Study the drawing (mm; zero at the part's minimum x, y, z) and answer. A direction names the side the tool comes from. Give positions to 0.01 mm unless a question says otherwise; leave off trailing zeros. Loops run counter-clockwise (first coordinate to the right, second up) from the corner with the lowest first, then second, coordinate; pieces in that order, holes last. Notation, with made-up numbers: (12, 37.25) - (54, 37.25) arc R31 cw to (54, 76.25) - close; hole circle Ø9 at (-35, -12.75). An arc over 180 degrees is marked (long way). Write item = value, one per line. Start each with the question number.
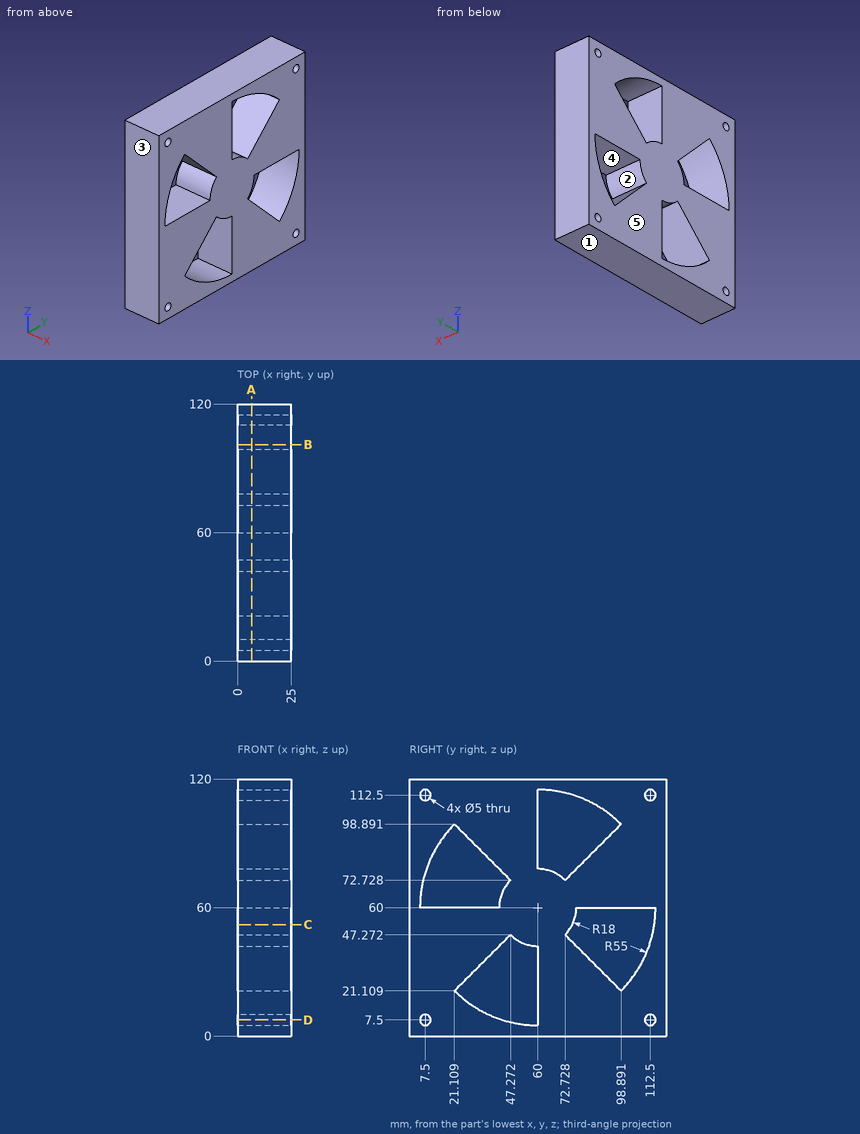
1. A tool of negligible diameter and unlimited length cuts with its end or side. For the marked faces 1 and 2, from which of +Z, -Z, +X, -X, +Y, -Y can it reach the whole face along a straight path? Write none if from no direction.
2. A cutting plane is placed at C-C on z = 52. Give the vertices of the cut face in (x, y) (1 decimal).
3. For a pull along Y with two mould halves and no side action, classify the marked faces 3, 4 and 5 as released by +Y, released by -Y, zero draft, split by the parting line, or undercut.
4. Consider line 1 along Y through (x, z) = (21, 40) (1 decimal); line 2 along Y through (x, z) = (3.5, 23.5); line 3 along Z through (x, y) = (9, 97.5). Determine where each line is inside the solid, lowest interval first. Write a range as [from, to].
5. A cutting plane is placed at B-B on y = 101. Give the vertices of the cut face in (x, z), and give its area (3 significant figures).
6. A cutting plane is placed at D-D on z = 7.5. Give the vertices of the cut face in (x, y), and give its area (3 significant figures).
7. A cutting plane is placed at A-A on x = 6.5. Give the number of separate pieces and of enclosed holes in the cut face, and give its area (3 significant figures).
8. Given P1, Ø4.5, axis at y = 112.5, z = 112.5, coming from the -X side, flat-ended and moving along its own axis, determine where the tip first touches the part or whether it passes through.
Reply:
q1.face_1 = -Z, +X, -X, +Y, -Y
q1.face_2 = +X, -X
q2.outline = (0, 0) - (25, 0) - (25, 76.1) - (0, 76.1) - close; (0, 114.4) - (25, 114.4) - (25, 120) - (0, 120) - close
q3.face_3 = released by -Y
q3.face_4 = undercut
q3.face_5 = zero draft
q4.line_1 = [0, 40], [60, 80], [111.2, 120]
q4.line_2 = [0, 23.5], [60, 96.5], [101.14, 120]
q4.line_3 = [0, 22.5], [60, 97.5], [100.23, 120]
q5.outline = (0, 0) - (25, 0) - (25, 23.34) - (0, 23.34) - close; (0, 60) - (25, 60) - (25, 120) - (0, 120) - close
q5.area = 2,080 mm^2
q6.outline = (0, 0) - (25, 0) - (25, 5) - (0, 5) - close; (0, 10) - (25, 10) - (25, 43.61) - (0, 43.61) - close; (0, 60) - (25, 60) - (25, 110) - (0, 110) - close; (0, 115) - (25, 115) - (25, 120) - (0, 120) - close
q6.area = 2,340 mm^2
q7.separate_pieces = 1
q7.enclosed_holes = 8
q7.area = 10,100 mm^2
q8.P1 = through
